from build123d import *

# Parameters (mm, degrees)
BOSS_EXTRUDE1_DEPTH = 36
CUT_EXTRUDE1_DEPTH  = 16.5
CUT_EXTRUDE2_DEPTH  = 10
SKETCH4_R           = 2.1
CUT_EXTRUDE3_DEPTH  = 60.338014797
SKETCH5_R           = 2.6
CUT_EXTRUDE4_DEPTH  = 60.338014797


with BuildPart() as part:
    # Sketch1 → Boss-Extrude1 (new, symmetric)
    with BuildSketch(Plane(origin=(0, 0, 0), x_dir=(1, 0, 0), z_dir=(0, 1, 0))):
        with BuildLine():
            Line((27.5, 0), (40, 0))
            Line((40, 0), (40, 25))
            Line((40, 25), (0, 25))
            Line((0, 25), (0, 0))
            Line((0, 0), (12.5, 0))
            ThreePointArc((12.5, 0), (20, 7.5), (27.5, 0))
        make_face()
    extrude(amount=BOSS_EXTRUDE1_DEPTH, both=True)

    # Sketch2 → Cut-Extrude1 (cut, symmetric)
    with BuildSketch(Plane(origin=(0, 0, 0), x_dir=(1, 0, 0), z_dir=(0, 1, 0))):
        with BuildLine():
            Line((8.5, 0), (31.5, 0))
            ThreePointArc((31.5, 0), (20, 11.5), (8.5, 0))
        make_face()
    extrude(amount=CUT_EXTRUDE1_DEPTH, both=True, mode=Mode.SUBTRACT)

    # Sketch3 → Cut-Extrude2 (cut)
    with BuildSketch(Plane(origin=(40, 0, 0), x_dir=(0, 0, -1), z_dir=(1, 0, 0))):
        with BuildLine():
            Line((25, 26.35), (25, 13.65))
            ThreePointArc((25, 13.65), (18.65, 20), (25, 26.35))
        make_face()
        with BuildLine():
            Line((25, -13.65), (25, -26.35))
            ThreePointArc((25, -26.35), (18.65, -20), (25, -13.65))
        make_face()
    extrude(amount=-CUT_EXTRUDE2_DEPTH, mode=Mode.SUBTRACT)

    # Sketch4 → Cut-Extrude3 (cut, through all)
    with BuildSketch(Plane(origin=(40, 0, 0), x_dir=(0, 0, -1), z_dir=(1, 0, 0))):
        with Locations((15, 14)):
            Circle(SKETCH4_R)
        with Locations((15, -14)):
            Circle(SKETCH4_R)
    extrude(amount=-CUT_EXTRUDE3_DEPTH, mode=Mode.SUBTRACT)

    # Sketch5 → Cut-Extrude4 (cut, through all)
    with BuildSketch(Plane.XY):
        with Locations((5, 31)):
            Circle(SKETCH5_R)
        with Locations((35, 31)):
            Circle(SKETCH5_R)
        with Locations((35, -31)):
            Circle(SKETCH5_R)
        with Locations((5, -31)):
            Circle(SKETCH5_R)
        with Locations((35, 0)):
            Circle(SKETCH5_R)
    extrude(amount=-CUT_EXTRUDE4_DEPTH, mode=Mode.SUBTRACT)


solid = part.part
For this review, take the finished solid that the model builds, in its own axes (mm). A direction names the side the tool comes from. Round coordinates to 2 decimals unless told otherwise and drop trailing zeros. Order: outer loops, then holes, each group sorted by start corner. A loop starts at its lowest first (then second) coordinate and runs counter-clockwise, first axis right, second up. Notation, with made-up numbers: (33, 34) -> (77, 34) arc R23 ccw to (77, 43) -> close; hole circle Ø2 at (70.25, -37.75). An arc over 180 degrees is marked (long way). Write item = value, one per line. Start each with the question number.
1) To check wall thickness, follow line 1 (Y direction, x = 30, z = -15); line 2 (Y direction, x = 11.5, z = -2.5); line 3 (Y direction, x = 35, z = -14). State the ranges of each line that lie inside material, in increasing order. Write a range as from..to.
2) Insertion check: pin 1 (4.5 mm diameter, centred on x = 35, y = 31, fed in from -Z); pin 2 (1.5 mm diameter, centred on x = 28, y = -6, fed in from +Z); pin 3 (3 mm diameter, centred on y = -21, z = -22.5, fed in from +X). Each pin has a flat end and moves straight along its axis. Give the tip position at first contact, or say it passes through.
3) Take a section at A-A on z = -15. State the section outline as (x, y) points.
4) Tool access review of faces 5 (the face through (19.84, 26.39, -7.5)), 6 (the face through (35.07, -20.14, -18.65)): name each direction out of +Z, -Z, +X, -X, +Y, -Y from which nothing blocks a thin tool from reaching the whole face with its end or side.
5) Take a section at D-D on y = -31. State the section outline as (x, z) points.
6) Take a section at C-C on x = 5. State the section outline as (y, z) points, plus the area to 3 significant figures.
7) Take a section at B-B on y = 0. State the section outline as (x, z) points.
8) The part is to be moulded in two halves that separate along Y. For faces 1 (the face through (32, 1, 0)), 2 (the face through (20, -16.5, -8)), 3 (the face through (20.253, 0.231, -11.497)), 4 (the face through (20, 36, -13)), say which applies: +Y half, -Y half, draft (parallel to the pull), parting line (faces both ways), or undercut.
Verdict:
q1.line_1 = -36..-16.1, -11.9..11.9, 16.1..36
q1.line_2 = -36..-16.5, 16.5..36
q1.line_3 = -36..-33.6, -28.4..-15.85, -12.15..-2.6, 2.6..12.15, 15.85..28.4, 33.6..36
q2.pin_1 = through
q2.pin_2 = -7.46
q2.pin_3 = 30
q3.outline = (0, -36) -> (40, -36) -> (40, -16.1) -> (0, -16.1) -> close; (0, -11.9) -> (40, -11.9) -> (40, 11.9) -> (0, 11.9) -> close; (0, 16.1) -> (40, 16.1) -> (40, 36) -> (0, 36) -> close; hole circle Ø5.2 at (5, -31); hole circle Ø5.2 at (5, 31); hole circle Ø5.2 at (35, -31); hole circle Ø5.2 at (35, 0); hole circle Ø5.2 at (35, 31)
q4.face_5 = +Z, +Y, -Y
q4.face_6 = -Z, +X
q5.outline = (0, -25) -> (2.4, -25) -> (2.4, 0) -> (0, 0) -> close; (7.6, -25) -> (32.4, -25) -> (32.4, 0) -> (27.5, 0) arc R7.5 cw to (12.5, 0) -> (7.6, 0) -> close; (37.6, -25) -> (40, -25) -> (40, 0) -> (37.6, 0) -> close
q6.outline = (-36, -25) -> (-33.6, -25) -> (-33.6, 0) -> (-36, 0) -> close; (-28.4, -25) -> (28.4, -25) -> (28.4, 0) -> (-28.4, 0) -> close; (33.6, -25) -> (36, -25) -> (36, 0) -> (33.6, 0) -> close; hole circle Ø4.2 at (-14, -15); hole circle Ø4.2 at (14, -15)
q6.area = 1,510 mm2
q7.outline = (0, -25) -> (32.4, -25) -> (32.4, 0) -> (31.5, 0) arc R11.5 cw to (8.5, 0) -> (0, 0) -> close; (37.6, -25) -> (40, -25) -> (40, 0) -> (37.6, 0) -> close
q8.face_1 = draft
q8.face_2 = undercut
q8.face_3 = undercut
q8.face_4 = +Y half
